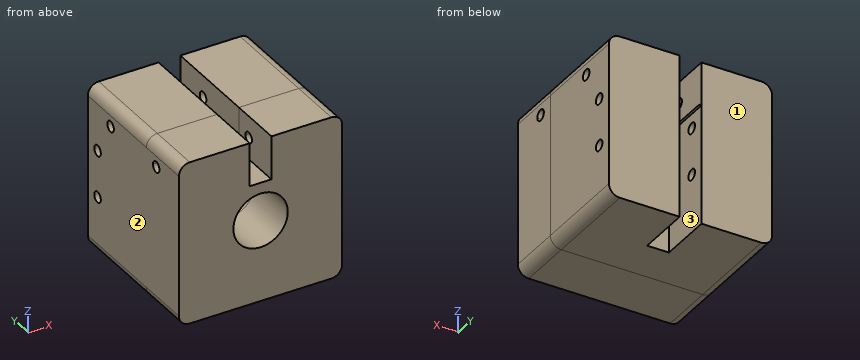
```python
from build123d import *

# Parameters (mm, degrees)
F0_W      = 75
F0_H      = 75
F1_DEPTH  = 45
F2_R      = 5
F3_R      = 12.5
F4_DEPTH  = 25
F6_DEPTH  = 20
F8_DEPTH  = 25
F10_DEPTH = 75.001
F11_DEPTH = 25
F12_R     = 2.5
F13_DEPTH = 75.001


with BuildPart() as f1:
    # F0 (on Front) → F1 (new body)
    with BuildSketch(Plane.XZ):
        with Locations((7.8840382397, -17.0557253063)):
            Rectangle(F0_W, F0_H)
    extrude(amount=F1_DEPTH)

    # F2
    f2_edges = [f1.edges().sort_by_distance(p)[0] for p in [
        (-29.615962, -22.5, 20.444275),
        (-29.615962, -22.5, -54.555725),
        (45.384038, -22.5, -54.555725),
        (45.384038, -22.5, 20.444275),
    ]]
    fillet(f2_edges, radius=F2_R)

    # F3 (on face) → F4 (cut)
    with BuildSketch(Plane.XZ.offset(45)):
        with Locations((7.8840382397, -17.0557253063)):
            Circle(F3_R)
    extrude(amount=-F4_DEPTH, mode=Mode.SUBTRACT)

    # F5 (on face) → F6 (cut)
    with BuildSketch(Plane.XY.offset(20.4442746937)):
        Polygon((7.8840382397, -25), (7.8840382397, 0), (2.8840382397, 0), (2.8840382397, -45), (7.8840382397, -45), align=None)
        Polygon((12.8840382397, 0), (7.8840382397, 0), (7.8840382397, -25), (7.8840382397, -45), (12.8840382397, -45), align=None)
    extrude(amount=-F6_DEPTH, mode=Mode.SUBTRACT)

    # F7 (on face) → F8 (cut)
    with BuildSketch(Plane.XZ):
        Polygon((12.8703957796, 0.5023097037), (2.8703957796, 0.4370668321), (2.8703957796, -54.635066539), (12.8703957796, -54.635066539), align=None)
    extrude(amount=F8_DEPTH, mode=Mode.SUBTRACT)

    # F9 (on face) → F10 (cut, through all)
    with BuildSketch(Plane(origin=(-29.6159617603, 0, 0), x_dir=(0, -1, 0), z_dir=(-1, 0, 0))):
        with BuildLine():
            ThreePointArc((10, -27.7557253063), (7.5, -25.2557253063), (5, -27.7557253063))
            ThreePointArc((5, -27.7557253063), (7.5, -30.2557253063), (10, -27.7557253063))
        make_face()
        with BuildLine():
            ThreePointArc((10, -6.1557253063), (7.5, -3.6557253063), (5, -6.1557253063))
            ThreePointArc((5, -6.1557253063), (7.5, -8.6557253063), (10, -6.1557253063))
        make_face()
    extrude(amount=-F10_DEPTH, mode=Mode.SUBTRACT)

    # F11 (add): a face of the model
    f11_faces = [f1.faces().sort_by_distance(p)[0] for p in [
        (43.1695721457, -45, -52.3412592122),
    ]]
    extrude(f11_faces, amount=F11_DEPTH)

    # F12 (on face) → F13 (cut, through all)
    with BuildSketch(Plane(origin=(-29.6159617603, 0, 0), x_dir=(0, -1, 0), z_dir=(-1, 0, 0))):
        with BuildLine():
            ThreePointArc((55, 10.4442746937), (54.267766953, 12.2120416467), (52.5, 12.9442746937))
            Line((52.5, 12.9442746937), (52.5, 10.4442746937))
            Line((52.5, 10.4442746937), (50, 10.4442746937))
            ThreePointArc((50, 10.4442746937), (52.5, 7.9442746937), (55, 10.4442746937))
        make_face()
        with Locations((17.5, 10.4442746937)):
            Circle(F12_R)
        with BuildLine():
            Line((52.5, 10.4442746937), (52.5, 12.9442746937))
            ThreePointArc((52.5, 12.9442746937), (50.732233047, 12.2120416467), (50, 10.4442746937))
            Line((50, 10.4442746937), (52.5, 10.4442746937))
        make_face()
    extrude(amount=-F13_DEPTH, mode=Mode.SUBTRACT)


solid = f1.part
```
Check sheet for the modelled part. Datum: model origin and axes. Units: mm. Face numbers are marked on the shaded views. Round coordinates to 2 decimals unless told otherwise and drop trailing zeros. Order: outer loops, then holes, each group sorted by start corner. A loop starts at its lowest first (then second) coordinate and runs counter-clockwise, first axis right, second up. Notation, with made-up numbers: M 63.5,-4.5 L 110.5,-4.5 A28 ccw 110.5,20.5 Z; hole C -7.5,58.5 d3. An arc over 180 degrees is marked long. Answer in a Markdown table with one row per item.
(1) Section check A-A on y = -17.5. Give the number of separate pieces and of enclosed holes in the cut face, plus the area to 3 significant figures.
Findings:
| item | result |
|---|---|
| separate pieces | 4 |
| enclosed holes | 0 |
| area | 4,530 mm^2 |
(2) Gauge pin test, flat ends, axial feed: pin 1 (4 mm diameter, centred on y = -7.5, z = -27.76, fed in from -X); pin 2 (15 mm diameter, centred on x = 7.88, z = -17.06, fed in from -Y). Record the tip position at first contact, or that the pin passes through.
Findings:
| item | result |
|---|---|
| pin 1 | passes through |
| pin 2 | stops at y = -20 |
(3) Section check D-D on z = -7.5. Record the boundary of the cut face in (x, y).
Findings:
| item | result |
|---|---|
| outline | M -29.62,-70 L -0.17,-70 L -0.17,-20 L 2.87,-20 L 2.87,-9.61 L -29.62,-9.61 Z; M -29.62,-5.39 L 2.87,-5.39 L 2.87,0 L -29.62,0 Z; M 12.87,-20 L 15.94,-20 L 15.94,-70 L 45.38,-70 L 45.38,-9.61 L 12.87,-9.61 Z; M 12.87,-5.39 L 45.38,-5.39 L 45.38,0 L 12.87,0 Z |
(4) Draft check along X on the marked faces 1, 2 and 3. Enter one of: +X half, -X half, draft (parallel to the pull), parting line (faces both ways), or undercut.
Findings:
| item | result |
|---|---|
| face 1 | draft |
| face 2 | -X half |
| face 3 | undercut |
(5) Section check C-C on x = 5.5. Record the boundary of the cut face in (y, z), plus the area to 3 significant figures.
Findings:
| item | result |
|---|---|
| outline | M -70,-54.56 L -25,-54.56 L -25,-29.33 L -70,-29.33 Z; M -70,-4.79 L -25,-4.79 L -25,0.44 L -70,0.44 Z |
| area | 1,370 mm^2 |
(6) Material ranges on line 1 along Z through (x, y) = (-22.5, -7.5); line 2 along X through (y, z) = (-21, 12.5); line 3 along Z through (x, y) = (8, -31), recorded low to high. Write a range as from..to.
Findings:
| item | result |
|---|---|
| line 1 | z = -54.56..-30.26, -25.26..-8.66, -3.66..20.44 |
| line 2 | x = -29.62..2.88, 12.88..45.38 |
| line 3 | z = -54.56..-29.56, -4.56..0.44 |
